from build123d import *

# Parameters (mm, degrees)
SKETCH_3_R                   = 6.5
EXTRUDE_1_DEPTH              = 5
SKETCH_4_R                   = 5
EXTRUDE_2_DEPTH              = 20
SKETCH_6_W                   = 25
SKETCH_6_H                   = 25
SKETCH_6_W_2                 = 24
SKETCH_6_H_2                 = 6.75
CUT_EXTRUDE_1_DEPTH          = 25
CUT_EXTRUDE_3_DEPTH          = 42.740268327
CUT_EXTRUDE_3_DEPTH_BACK     = 42.740268327
SKETCH_10_R                  = 3
HOLE_WIZARD_M6_1_D           = 5
HOLE_WIZARD_M6_1_DEPTH       = 15
HOLE_WIZARD_M6_1_CSINK_D     = 6.05
HOLE_WIZARD_M6_1_CSINK_ANGLE = 90
HOLE_WIZARD_M6_1_TIP         = 1.502151548
SKETCH_16_R                  = 20
SKETCH_16_W                  = 25
SKETCH_16_H                  = 9
CUT_EXTRUDE_4_DEPTH          = 24.286262044


with BuildPart() as part:
    # 草图3 → 凸台-拉伸1 (new body)
    with BuildSketch(Plane.XY):
        Circle(SKETCH_3_R)
    extrude(amount=EXTRUDE_1_DEPTH)

    # 草图4 → 凸台-拉伸2 (add)
    with BuildSketch(Plane.XY.offset(5)):
        Circle(SKETCH_4_R)
    extrude(amount=EXTRUDE_2_DEPTH)

    # 草图5 → 旋转4 (revolve)
    with BuildSketch(Plane(origin=(0, 0, 0), x_dir=(1, 0, 0), z_dir=(0, 1, 0))):
        with BuildLine():
            Line((0, -20), (0, -40))
            ThreePointArc((0, -40), (-10, -30), (0, -20))
        make_face()
    revolve(axis=Axis((0, 0, 0), (0, 0, 1)))

    # 草图6 → 切除-拉伸1 (cut)
    with BuildSketch(Plane.XY.offset(20)):
        Rectangle(SKETCH_6_W, SKETCH_6_H)
        Rectangle(SKETCH_6_W_2, SKETCH_6_H_2, mode=Mode.SUBTRACT)
    extrude(amount=CUT_EXTRUDE_1_DEPTH, mode=Mode.SUBTRACT)

    # 草图8 → 旋转5 (revolve)
    with BuildSketch(Plane(origin=(0, 0, 0), x_dir=(1, 0, 0), z_dir=(0, 1, 0))):
        with BuildLine():
            Line((-6.35, -30), (6.35, -30))
            ThreePointArc((6.35, -30), (0, -36.35), (-6.35, -30))
        make_face()
    revolve(axis=Axis((-10, 0, 30), (1, 0, 0)))

    # 草图10 → 切除-拉伸3 (cut, two sides: drawn at the far end of the back side and taken through both)
    with BuildSketch(Plane(origin=(0, 0, 0), x_dir=(1, 0, 0), z_dir=(0, 1, 0)).offset(-CUT_EXTRUDE_3_DEPTH_BACK)):
        with Locations(Location((0, -30, 0), (0, 0, 180))):
            Circle(SKETCH_10_R)
    extrude(amount=CUT_EXTRUDE_3_DEPTH + CUT_EXTRUDE_3_DEPTH_BACK, mode=Mode.SUBTRACT)

    # M6 螺纹孔1
    with Locations(Plane(origin=(0, 0, 0), x_dir=(-1, 0, 0), z_dir=(0, 0, -1))):
        with Locations((0, 0)):
            CounterSinkHole(HOLE_WIZARD_M6_1_D / 2, HOLE_WIZARD_M6_1_CSINK_D / 2, depth=HOLE_WIZARD_M6_1_DEPTH, counter_sink_angle=HOLE_WIZARD_M6_1_CSINK_ANGLE)
            with Locations((0, 0, -(HOLE_WIZARD_M6_1_DEPTH + HOLE_WIZARD_M6_1_TIP / 2))):  # 118° drill point
                Cone(0, HOLE_WIZARD_M6_1_D / 2, HOLE_WIZARD_M6_1_TIP, mode=Mode.SUBTRACT)

    # 草图16 → 切除-拉伸4 (cut, through all)
    with BuildSketch(Plane.XY.offset(20)):
        Circle(SKETCH_16_R)
        Rectangle(SKETCH_16_W, SKETCH_16_H, mode=Mode.SUBTRACT)
    extrude(amount=CUT_EXTRUDE_4_DEPTH, mode=Mode.SUBTRACT)


solid = part.part
Verification items for the finished model (mm, model axes). A direction names the side the tool comes from. Give positions to 0.01 mm unless a question says otherwise; leave off trailing zeros. Write each loop counter-clockwise with the first axis right and the second up, starting at its lowest first coordinate (ties: lowest second). Pieces come first, ordered by that corner, then holes.
(1) Gauge pin test, flat ends, axial feed: pin 1 (1.5 mm diameter, centred on x = 0, z = 21, fed in from +Y) (3 decimals); pin 2 (10 mm diameter, centred on x = -3, z = 23.5, fed in from +Y); pin 3 (1.3 mm diameter, centred on x = 2, y = 4.5, fed in from +Z). Record the tip position at first contact, or that the pin passes through.
(2) Material ranges on line 1 (Z direction, x = -2.5, y = 4); line 2 (X direction, y = 0, z = 5.5); line 3 (Z direction, x = 0, y = -2.25), recorded low to high.
(3) Cross-section at D-D (z = 14). Enter the section's corners in (x, y), plus the area to 3 significant figures.
(4) Mould release check, pull along X, two halves, no side actions. Record for faces 1 (the face through (0, 4, 20)), 2 (the face through (-0.54, -2.44, 7.86)), 3 (the face through (-1.08, -4.88, 13.06)): +X half, -X half, draft (parallel to the pull), parting line (faces both ways), or undercut.
(5) Cross-section at A-A (z = 30). Enter the section's corners in (x, y) (3 decimals), plus the area to 3 significant figures.
(6) Cross-section at B-B (z = 3.5). Enter the section's corners in (x, y), plus the area to 3 significant figures.
(7) Cross-section at C-C (x = 8.5). Enter the section's corners in (y, z) (3 decimals).
(8) Access from +Z, -Z, +X, -X, +Y, -Y to the whole of each face (thin tool, end or side, straight path). Record for faces 4 (the face through (4, 3.375, 34)), 5 (the face through (3, -4.5, 31)), 6 (the face through (2, -5, 5)), 7 (the face through (4, -3.375, 34)).
Worked out:
1. pin 1: stops at y = 3.375
1. pin 2: stops at y = 5
1. pin 3: stops at z = 34.7
2. line 1: z = 0 to 20, 25.75 to 28.34, 31.66 to 34.25
2. line 2: x = -5 to -2.5, 2.5 to 5
2. line 3: z = 15.15 to 27, 33 to 39.74
3. outline: circle Ø10 at (0, 0); hole circle Ø5 at (0, 0)
3. area: 58.9 mm2
4. face 1: draft
4. face 2: undercut
4. face 3: parting line
5. outline: (-9.413, -3.375) - (-5.379, -3.375) arc R6.35 ccw to (-4.48, -4.5) - (-3, -4.5) - (-3, 4.5) - (-4.48, 4.5) arc R6.35 ccw to (-5.379, 3.375) - (-9.413, 3.375) arc R10 ccw to start; (3, -4.5) - (4.48, -4.5) arc R6.35 ccw to (5.379, -3.375) - (9.413, -3.375) arc R10 ccw to (9.413, 3.375) - (5.379, 3.375) arc R6.35 ccw to (4.48, 4.5) - (3, 4.5) - close
5. area: 101 mm2
6. outline: circle Ø13 at (0, 0); hole circle Ø5 at (0, 0)
6. area: 113 mm2
7. outline: (-3.375, 25.955) arc R5.268 ccw to (3.375, 25.955) - (3.375, 34.045) arc R5.268 ccw to (-3.375, 34.045) - close
8. face 4: +Y
8. face 5: +Z, +X, -X, -Y
8. face 6: none
8. face 7: -Y
